from build123d import *

# Parameters (mm, degrees)
SKETCH1_W           = 394.926652775
SKETCH1_H           = 202.769674437
BOSS_EXTRUDE1_DEPTH = 333
SHELL5_T            = -10
BOSS_EXTRUDE2_DEPTH = 7
SKETCH19_R          = 24.92303726
CUT_EXTRUDE1_DEPTH  = 14
BOSS_EXTRUDE3_DEPTH = 7
SKETCH23_R          = 24.92303726
CUT_EXTRUDE2_DEPTH  = 14


with BuildPart() as part:
    # Sketch1 → Boss-Extrude1 (new body)
    with BuildSketch(Plane.XY):
        with Locations((197.463326388, 101.384837219)):
            Rectangle(SKETCH1_W, SKETCH1_H)
    extrude(amount=BOSS_EXTRUDE1_DEPTH)

    # Shell5
    shell5_openings = [part.faces().sort_by_distance(p)[0] for p in [
        (197.463326387, 101.384837219, 333),
    ]]
    offset(amount=SHELL5_T, openings=shell5_openings, kind=Kind.INTERSECTION)

    # Sketch18 → Boss-Extrude2 (add, symmetric)
    with BuildSketch(Plane.XY.offset(166.5)):
        with BuildLine():
            Line((10, 128.355944405), (81.814439739, 128.355944405))
            ThreePointArc((81.814439739, 128.355944405), (117.012291579, 93.158092565), (81.814439739, 57.960240724))
            Line((81.814439739, 57.960240724), (10, 57.960240724))
            Line((10, 57.960240724), (10, 128.355944405))
        make_face()
    extrude(amount=BOSS_EXTRUDE2_DEPTH, both=True)

    # Sketch19 → Cut-Extrude1 (cut)
    with BuildSketch(Plane.XY.offset(173.5)):
        with Locations((81.814439739, 93.158092565)):
            Circle(SKETCH19_R)
    extrude(amount=-CUT_EXTRUDE1_DEPTH, mode=Mode.SUBTRACT)

    # Sketch22 → Boss-Extrude3 (add, symmetric)
    with BuildSketch(Plane.XY.offset(166.5)):
        with BuildLine():
            Line((384.926652775, 128.355944405), (291.108955259, 128.355944405))
            ThreePointArc((291.108955259, 128.355944405), (256.621992249, 93.868981396), (291.108955259, 59.382018386))
            Line((291.108955259, 59.382018386), (384.926652775, 59.382018386))
            Line((384.926652775, 59.382018386), (384.926652775, 128.355944405))
        make_face()
    extrude(amount=BOSS_EXTRUDE3_DEPTH, both=True)

    # Sketch23 → Cut-Extrude2 (cut)
    with BuildSketch(Plane.XY.offset(173.5)):
        with Locations((291.108955259, 93.868981396)):
            Circle(SKETCH23_R)
    extrude(amount=-CUT_EXTRUDE2_DEPTH, mode=Mode.SUBTRACT)


solid = part.part
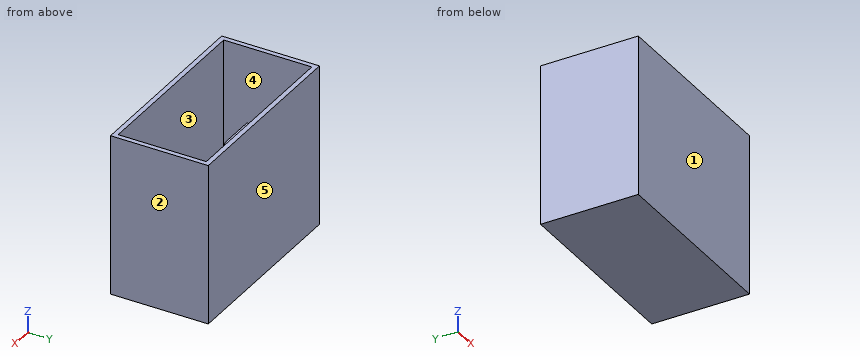
CAD build for the part. Positions are in the model's coordinates, mm. Face numbers are marked on the shaded views. A direction names the side the tool comes from. Give positions to 0.01 mm unless a question says otherwise; leave off trailing zeros. Loops run counter-clockwise (first coordinate to the right, second up) from the corner with the lowest first, then second, coordinate; pieces in that order, holes last. Notation, with made-up numbers: M -2.5,22 L 51.5,22 A17 cw 51.5,34 Z; hole C -32,-30.75 d10. An arc over 180 degrees is marked long. One line per question, with ' | ' between items. Start each with the question number.
1. Saw through at A-A on x = 33. Give the cut face in (y, z).
2. Flat gauge pins, fed straight in: pin 1 (4 mm diameter, centred on x = 289.5, y = 111.5, fed in from -Z); pin 2 (12 mm diameter, centred on x = 261, y = 78.5, fed in from +Z). Where does each tip first touch, or does it go through?
3. Saw through at B-B on z = 213.5. Give the cut face in (x, y), plus the area to 3 significant figures.
4. Two-plate mould, pull along Y, no slides. Class the marked faces 1, 2 and 3: pulls with the +Y half, pulls with the -Y half, needs draft (parallel to the pull), parting line crosses it, or undercut.
5. 3-axis set-ups, long thin cutter, end or side, ignore diameter. For the marked faces 4 and 5: which of +Z, -Z, +X, -X, +Y, -Y reach the whole face in a straight line?
6. Probe L1, parallel to X at y = 127.5, z = 92; L2, parallel to Y at x = 322.5, z = 164; L3, parallel to Y at x = 254, z = 81. List the from-to ranges inside material, lowest first. Write a range as from..to.
7. Saw through at C-C on y = 111. Give the cut face in (x, z), plus the area to 3 significant figures.
8. Saw through at D-D on x = 284. Give the cut face in (y, z), plus the area to 3 significant figures.
Result sheet:
1) outline: M 0,0 L 202.77,0 L 202.77,333 L 192.77,333 L 192.77,10 L 10,10 L 10,333 L 0,333 Z; M 57.96,159.5 L 128.36,159.5 L 128.36,173.5 L 57.96,173.5 Z
2) pin 1: stops at z = 0 | pin 2: stops at z = 173.5
3) outline: M 0,0 L 394.93,0 L 394.93,202.77 L 0,202.77 Z; hole M 10,10 L 384.93,10 L 384.93,192.77 L 10,192.77 Z | area: 11,600 mm^2
4) face 1: pulls with the -Y half | face 2: needs draft | face 3: undercut
5) face 4: none | face 5: +Z, -Z, +X, -X, +Y
6) L1: x = 0..10, 384.93..394.93 | L2: y = 0..10, 59.38..128.36, 192.77..202.77 | L3: y = 0..10, 192.77..202.77
7) outline: M 0,0 L 394.93,0 L 394.93,333 L 384.93,333 L 384.93,173.5 L 309.21,173.5 L 309.21,159.5 L 384.93,159.5 L 384.93,10 L 10,10 L 10,159.5 L 64.41,159.5 L 64.41,173.5 L 10,173.5 L 10,333 L 0,333 Z; M 99.22,159.5 L 112.16,159.5 L 112.16,173.5 L 99.22,173.5 Z; M 261.18,159.5 L 273.01,159.5 L 273.01,173.5 L 261.18,173.5 Z | area: 12,600 mm^2
8) outline: M 0,0 L 202.77,0 L 202.77,333 L 192.77,333 L 192.77,10 L 10,10 L 10,333 L 0,333 Z; M 60.12,159.5 L 69.98,159.5 L 69.98,173.5 L 60.12,173.5 Z; M 117.76,159.5 L 127.62,159.5 L 127.62,173.5 L 117.76,173.5 Z | area: 8,760 mm^2
